Check sheet for the modelled part. Datum: model origin and axes. Units: mm. Face numbers are marked on the shaded views. A direction names the side the tool comes from. Give positions to 0.01 mm unless a question says otherwise; leave off trailing zeros. Write each loop counter-clockwise with the first axis right and the second up, starting at its lowest first coordinate (ties: lowest second). Pieces come first, ordered by that corner, then holes. Notation, with made-up numbers: (63.25, -34.75) -> (80.25, -34.75) arc R16 cw to (80.25, -6.75) -> close; hole circle Ø1 at (16, -39). An arc over 180 degrees is marked (long way). Return JSON: item names as keys, results as strings.
from build123d import *

# Parameters (mm, degrees)
CBORE_FOR_M3_SHCS1_D           = 3.4
CBORE_FOR_M3_SHCS1_CBORE_D     = 6.5
CBORE_FOR_M3_SHCS1_CBORE_DEPTH = 40


with BuildPart() as part:
    # Sketch2 → Revolve1 (revolve)
    with BuildSketch(Plane(origin=(0, 0, 0), x_dir=(-1, 0, 0), z_dir=(0, -1, 0)), mode=Mode.PRIVATE) as revolve1_sk:
        Polygon((5, 0), (5, -50), (24, -50), (15, -44.803847577), (15, -5.196152423), (24, 0), align=None)
    revolve(revolve1_sk.sketch.rotate(Axis((0, 0, 0), (0, 0, 1)), 270), axis=Axis((0, 0, 0), (0, 0, 1)))

    # CBORE for M3 SHCS1 (through all)
    with Locations(Plane.XY.offset(50)):
        with Locations((0, -9), (0, 9)):
            CounterBoreHole(CBORE_FOR_M3_SHCS1_D / 2, CBORE_FOR_M3_SHCS1_CBORE_D / 2, CBORE_FOR_M3_SHCS1_CBORE_DEPTH)


solid = part.part
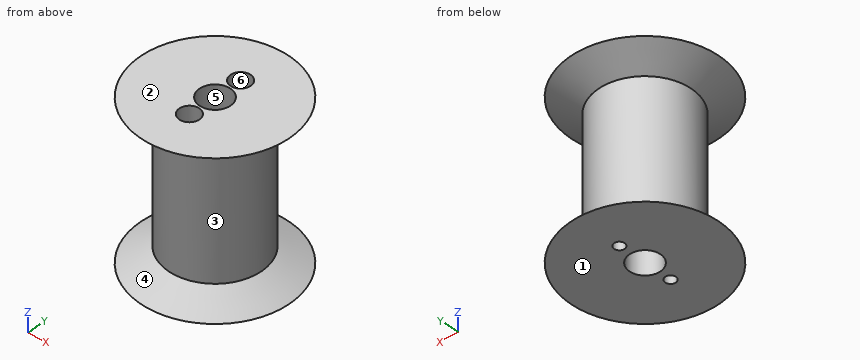
(1) Cross-section at D-D on z = 12.5. Enter the section's corners in (x, y), then the cut area to 3 significant figures.
Reply:
{"outline": "circle Ø30 at (0, 0); hole circle Ø10 at (0, 0); hole circle Ø6.5 at (0, -9); hole circle Ø6.5 at (0, 9)", "area": "562 mm^2"}
(2) Depth check by flat-ended pin: pin 1 Ø5 at (y, z) = (-0.5, 14) entering from -X; pin 2 Ø1.5 at (y, z) = (-7, 19) entering from +X; pin 3 Ø2 at (x, z) = (0, 29) entering from +Y. Enter the tip coordinate at first touch or a pass-through.
Reply:
{"pin 1": "x = -15", "pin 2": "x = 13.64", "pin 3": "y = 15"}
(3) Release check for a two-part mould opening along Z. For the marked faces 1, 2 and 3 record: pulls with the +Z half, pulls with the -Z half, needs draft (parallel to the pull), parting line crosses it, or undercut.
Reply:
{"face 1": "pulls with the -Z half", "face 2": "pulls with the +Z half", "face 3": "undercut"}
(4) Cross-section at C-C on z = 7.5. Enter the section's corners in (x, y).
Reply:
{"outline": "circle Ø30 at (0, 0); hole circle Ø10 at (0, 0); hole circle Ø3.4 at (0, -9); hole circle Ø3.4 at (0, 9)"}
(5) Set-up check for the marked faces 4, 5 and 6: record each of +Z, -Z, +X, -X, +Y, -Y from which the full face is reachable in a straight line by a thin tool's end or side.
Reply:
{"face 4": "none", "face 5": "+Z, -Z", "face 6": "+Z"}
(6) Cross-section at A-A on y = 0. Enter the section's corners in (x, z), then the cut area to 3 significant figures.
Reply:
{"outline": "(-24, 0) -> (-5, 0) -> (-5, 50) -> (-24, 50) -> (-15, 44.8) -> (-15, 5.2) -> close; (5, 0) -> (24, 0) -> (15, 5.2) -> (15, 44.8) -> (24, 50) -> (5, 50) -> close", "area": "1,090 mm^2"}
(7) Cross-section at B-B on x = 0. Enter the section's corners in (y, z), then the cut area to 3 significant figures.
Reply:
{"outline": "(-24, 0) -> (-10.7, 0) -> (-10.7, 10) -> (-12.25, 10) -> (-12.25, 50) -> (-24, 50) -> (-15, 44.8) -> (-15, 5.2) -> close; (-7.3, 0) -> (-5, 0) -> (-5, 50) -> (-5.75, 50) -> (-5.75, 10) -> (-7.3, 10) -> close; (5, 0) -> (7.3, 0) -> (7.3, 10) -> (5.75, 10) -> (5.75, 50) -> (5, 50) -> close; (10.7, 0) -> (24, 0) -> (15, 5.2) -> (15, 44.8) -> (24, 50) -> (12.25, 50) -> (12.25, 10) -> (10.7, 10) -> close", "area": "506 mm^2"}
(8) Thickness scan on L1, parallel to X at y = 0, z = 13.5; L2, parallel to Z at x = -19.5, y = 1; L3, parallel to X at y = 9.5, z = 21.5. Record the ranges inside material, lowest first.
Reply:
{"L1": "-15 to -5, 5 to 15", "L2": "0 to 2.58, 47.42 to 50", "L3": "-11.61 to -3.21, 3.21 to 11.61"}
